Read the model definition and answer for the solid it produces. Units are mm, in the model's axes. Give positions to 0.01 mm unless a question says otherwise; leave off trailing zeros. Order: outer loops, then holes, each group sorted by start corner. A loop starts at its lowest first (then second) coordinate and runs counter-clockwise, first axis right, second up. Notation, with made-up numbers: (8.25, 25.5) - (57.25, 25.5) arc R26 ccw to (57.25, 59.5) - close; hole circle Ø10 at (-37, 55.5). An arc over 180 degrees is marked (long way). Write each question's results on one line, items separated by ' | '.
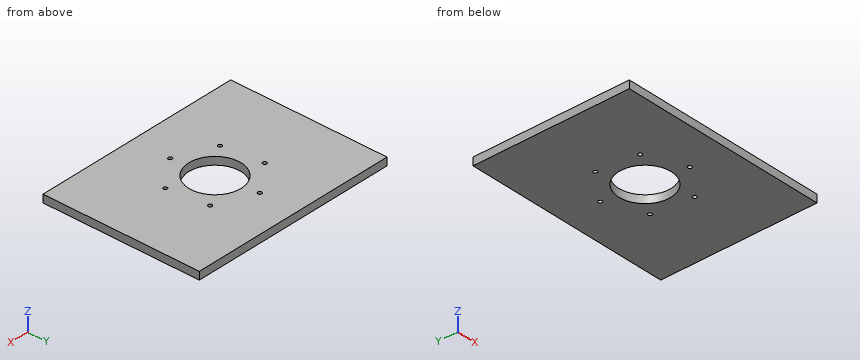
Autodesk Inventor part; units mm, degrees
ref_plane "YZ Plane" through (0, 0, 0) normal (1, 0, 0) x (0, 1, 0)
ref_plane "XZ Plane" through (0, 0, 0) normal (0, 1, 0) x (-1, 0, 0)
ref_plane "XY Plane" through (0, 0, 0) normal (0, 0, 1) x (1, 0, 0)
sketch "Sketch1" plane through (0, 0, 0) normal (0, 0, 1) x (1, 0, 0)
  line L0 (-80, -60) -> (80, -60)
  line L1 (80, -60) -> (80, 60)
  line L2 (80, 60) -> (-80, 60)
  line L3 (-80, 60) -> (-80, -60)
  line L4 (-80, -60) -> (80, 60) construction
  line L5 (80, -60) -> (-80, 60) construction
  circle A0 centre (0, 0) radius 20
  point P0 (25, 18.75)
  dimension "d0" = 160
  dimension "d1" = 120
  dimension "d2" = 40
  dimension "d5" = 25
extrude "Extrusion1" add sketch "Sketch1" along normal blind 6
hole "Hole1" at (25, 18.75, 0) direction (0, 0, 1) diameter 3 end through all
pattern_circular "Circular Pattern1" count 6 over 360 about axis through (0, 0, 0) along (0, 0, 1) of "Hole1"
properties part number "base_plate" material "Plywood, Finish"
(1) Section C-C (z = 2.15) is taken. Give the vertices of the cut face in (x, y).
Conclusion:
outline: (-80, -60) - (80, -60) - (80, 60) - (-80, 60) - close; hole circle Ø3 at (-28.74, 12.28); hole circle Ø3 at (-25, -18.75); hole circle Ø40 at (0, 0); hole circle Ø3 at (-3.74, 31.03); hole circle Ø3 at (3.74, -31.03); hole circle Ø3 at (25, 18.75); hole circle Ø3 at (28.74, -12.28)
(2) Section A-A (x = 0) is taken. Give the vertices of the cut face in (y, z), plus the area to 3 significant figures.
Conclusion:
outline: (-60, 0) - (-20, 0) - (-20, 6) - (-60, 6) - close; (20, 0) - (60, 0) - (60, 6) - (20, 6) - close | area: 480 mm^2
(3) Consider probe 1 along Y at (x, z) = (-1, 4.35); probe 2 along Y at (x, z) = (3, 1.8); probe 3 along Y at (x, z) = (-2.5, 0.95). Determine where each line is inside the solid, lowest interval first. Write a range as [from, to].
Conclusion:
probe 1: [-60, -19.97], [19.97, 60] | probe 2: [-60, -32.33], [-29.72, -19.77], [19.77, 60] | probe 3: [-60, -19.84], [19.84, 30.18], [31.87, 60]
(4) This flat-tipped pin is pushed along its axis until it touches: pin 1 (2.5 mm diameter, centred on x = -3.74, y = 31.03, fed in from +Z). Where does it stop, or does it pass through?
Conclusion:
pin 1: through
(5) Section B-B (y = 0) is taken. Give the vertices of the cut face in (x, z), plus the area to 3 significant figures.
Conclusion:
outline: (-80, 0) - (-20, 0) - (-20, 6) - (-80, 6) - close; (20, 0) - (80, 0) - (80, 6) - (20, 6) - close | area: 720 mm^2
